Autodesk Inventor part; units mm, degrees
ref_plane "YZ Plane" through (0, 0, 0) normal (1, 0, 0) x (0, 1, 0)
ref_plane "XZ Plane" through (0, 0, 0) normal (0, 1, 0) x (-1, 0, 0)
ref_plane "XY Plane" through (0, 0, 0) normal (0, 0, 1) x (1, 0, 0)
sketch "Sketch1" plane through (0, 0, 0) normal (0, 0, 1) x (1, 0, 0)
  line L0 (-3.1319, 102.9805) -> (141.8681, 102.9805)
  line L1 (144.3681, 100.4805) -> (144.3681, 95.4805)
  line L2 (141.8681, 92.9805) -> (-3.1319, 92.9805)
  line L3 (-5.6319, 95.4805) -> (-5.6319, 100.4805)
  line L4 (141.8681, 102.9805) -> (144.3681, 100.4805)
  line L5 (-3.1319, 102.9805) -> (-5.6319, 100.4805)
  line L6 (-5.6319, 95.4805) -> (-3.1319, 92.9805)
  line L7 (141.8681, 92.9805) -> (144.3681, 95.4805)
  line L8 (69.3681, 92.9805) -> (69.3681, 132.9805) construction
  line L9 (84.3681, 102.9805) -> (54.3681, 102.9805)
  line L10 (54.3681, 102.9805) -> (54.3681, 112.9805)
  line L11 (64.3681, 122.9805) -> (74.3681, 122.9805)
  line L12 (84.3681, 112.9805) -> (84.3681, 102.9805)
  line L13 (74.3681, 122.9805) -> (84.3681, 112.9805)
  line L14 (54.3681, 112.9805) -> (64.3681, 122.9805)
  circle A0 centre (69.3681, 107.9805) radius 12.5 construction
  point P0 (0, 0)
  point P1 (-5.6319, 102.9805)
  point P2 (144.3681, 92.9805)
  point P3 (144.3681, 102.9805)
  point P4 (-5.6319, 92.9805)
  point P5 (54.3681, 122.9805)
  point P6 (84.3681, 122.9805)
  dimension "d0" = 150
  dimension "d1" = 10
  dimension "d2" = 2.5
  dimension "d3" = 2.5
  dimension "d4" = 2.5
  dimension "d5" = 2.5
  dimension "d6" = 2.5
  dimension "d7" = 2.5
  dimension "d8" = 2.5
  dimension "d9" = 2.5
  dimension "d12" = 40
  dimension "d13" = 30
  dimension "d14" = 20
  dimension "d15" = 15
  dimension "d16" = 10
  dimension "d17" = 10
  dimension "d18" = 10
  dimension "d19" = 10
  dimension "d20" = 25
extrude "Extrusion1" add sketch "Sketch1" along normal blind 7
sketch "Sketch2" plane through (0, 0, 7) normal (0, 0, 1) x (1, 0, 0)
  line L0 (74.3681, 122.9805) -> (64.3681, 122.9805) construction
  line L1 (69.3681, 122.9805) -> (69.3681, 92.9805) construction
  line L2 (-3.1319, 92.9805) -> (141.8681, 92.9805) construction
  line L3 (-5.6319, 100.4805) -> (-5.6319, 95.4805) construction
  point P0 (0, 0)
  point P1 (-0.6319, 97.9805)
  point P2 (139.3681, 97.9805)
  dimension "d21" = 5
hole "Hole1" at (-0.6319, 97.9805, 7) at (139.3681, 97.9805, 7) direction (0, 0, -1) diameter 4 end through all
properties part number "Lever" material "MDF Medium Density Fiberboard"
Could you check a few things on this model? Use its own coordinates, in mm. A direction names the side the tool comes from. Give positions to 0.01 mm unless a question says otherwise; leave off trailing zeros. Write each loop counter-clockwise with the first axis right and the second up, starting at its lowest first coordinate (ties: lowest second). Pieces come first, ordered by that corner, then holes. Notation, with made-up numbers: (6.5, -6) -> (27.5, -6) arc R19 cw to (27.5, 1) -> close; hole circle Ø9 at (-3.5, -18). An arc over 180 degrees is marked (long way). Answer as CSV lines item,"result". Start each with the question number.
(1) If we section it at C-C, the plane x = 134: Write out the boundary of the cut face in (y, z).
(2) If we section it at B-B, the plane z = 5.75: Write out the boundary of the cut face in (x, y), and give its area (3 significant figures).
(3) I'm going to push flat-ended pins straight in: pin 1 Ø3 at (y, z) = (118, 2) entering from +X; pin 2 Ø1 at (x, z) = (76.5, 3) entering from +Y; pin 3 Ø3.5 at (y, z) = (108, 4.5) entering from -X. Where does each tip first touch, or does it pass through?
(4) Which directions (+Z, -Z, +X, -X, +Y, -Y) give clear straight access to the entire face, cutting with the end or side of a thin tool? Please do faces 4 (the face through (54.368, 108, 3)), 5 (the face through (84.368, 108, 3)), 6 (the face through (70, 92.98, 3)).
(5) If we section it at A-A, the plane y = 97.5: Write out the boundary of the cut face in (x, z).
(6) If we mould it in two halves opening along Y, with no side actions, what happens to faces 1 (the face through (113, 102.98, 3)), 2 (the face through (-0.72, 99.98, 3.45)), 3 (the face through (143.1, 94.21, 3.45))? For each: +Y half, -Y half, draft (parallel to the pull), parting line (faces both ways), or undercut.
(7) Please list where these lines run through material, in increasing order: line 1 (X direction, y = 99, z = 5); line 2 (X direction, y = 96.75, z = 4.5); line 3 (X direction, y = 105.75, z = 4.5).
(8) If we section it at D-D, the plane y = 110: Write out the boundary of the cut face in (x, z), and give its area (3 significant figures).
Answer list:
1,outline,"(92.98, 0) -> (102.98, 0) -> (102.98, 7) -> (92.98, 7) -> close"
2,outline,"(-5.63, 95.48) -> (-3.13, 92.98) -> (141.87, 92.98) -> (144.37, 95.48) -> (144.37, 100.48) -> (141.87, 102.98) -> (84.37, 102.98) -> (84.37, 112.98) -> (74.37, 122.98) -> (64.37, 122.98) -> (54.37, 112.98) -> (54.37, 102.98) -> (-3.13, 102.98) -> (-5.63, 100.48) -> close; hole circle Ø4 at (-0.63, 97.98); hole circle Ø4 at (139.37, 97.98)"
2,area,"1,960 mm^2"
3,pin 1,"x = 80.85"
3,pin 2,"y = 121.35"
3,pin 3,"x = 54.37"
4,face 4,"+Z, -Z, -X, +Y"
4,face 5,"+Z, -Z, +X, +Y"
4,face 6,"+Z, -Z, +X, -X, -Y"
5,outline,"(-5.63, 0) -> (-2.57, 0) -> (-2.57, 7) -> (-5.63, 7) -> close; (1.31, 0) -> (137.43, 0) -> (137.43, 7) -> (1.31, 7) -> close; (141.31, 0) -> (144.37, 0) -> (144.37, 7) -> (141.31, 7) -> close"
6,face 1,"+Y half"
6,face 2,"undercut"
6,face 3,"-Y half"
7,line 1,"-5.63 to -2.35, 1.09 to 137.65, 141.09 to 144.37"
7,line 2,"-5.63 to -2.21, 0.94 to 137.79, 140.94 to 144.37"
7,line 3,"54.37 to 84.37"
8,outline,"(54.37, 0) -> (84.37, 0) -> (84.37, 7) -> (54.37, 7) -> close"
8,area,"210 mm^2"
